Read the model definition and answer for the solid it produces. Units are mm, in the model's axes. A direction names the side the tool comes from. Coordinates: 2 decimals unless noted, no trailing zeros. Order: outer loops, then holes, each group sorted by start corner. A loop starts at its lowest first (then second) coordinate and runs counter-clockwise, first axis right, second up.
Autodesk Inventor part; units mm, degrees
ref_plane "Work Plane1" through (0, 2.6, 0) normal (0, -1, 0) x (1, 0, 0)
ref_plane "YZ Plane" through (0, 0, 0) normal (1, 0, 0) x (0, 1, 0)
ref_plane "XZ Plane" through (0, 0, 0) normal (0, 1, 0) x (-1, 0, 0)
sketch "Sketch1" plane through (0, 0, 0) normal (0, 1, 0) x (-1, 0, 0)
  line L0 (4.7, 5.15) -> (-4.7, 5.15)
  line L1 (-4.7, 5.15) -> (-4.7, -5.15)
  line L2 (-4.7, -5.15) -> (4.7, -5.15)
  line L3 (4.7, -5.15) -> (4.7, 5.15)
  point P0 (0, 0)
  dimension "d0" = 9.4
  dimension "d1" = 4.7
  dimension "d2" = 10.3
  dimension "d3" = 5.15
extrude "Extrusion1" add sketch "Sketch1" along normal blind 4.7
chamfer "Chamfer1" distance 3.3 angle 15 1 edges at (0, 4.7, 5.15) measured on face at (-1.5667, 1.5667, 5.15)
chamfer "Chamfer2" distance 3.3 angle 15 1 edges at (4.7, 4.7, -0.4421) measured on face at (4.7, 3.1333, -2.0114)
chamfer "Chamfer3" distance 3.3 angle 15 1 edges at (-0.4421, 4.7, -5.15) measured on face at (-1.8614, 3.1333, -5.15)
chamfer "Chamfer4" distance 3.3 angle 15 1 edges at (-4.7, 4.7, 0) measured on face at (-4.7, 2.5, -1.4219)
sketch "Sketch2" plane through (0, 0, 0) normal (0, -1, 0) x (1, 0, 0)
  line L0 (4.7, 5.15) -> (4.7, -5.15)
  line L1 (11.3, -5.15) -> (11.3, 5.1662)
  line L2 (11.3, 5.1662) -> (4.7, 5.1662)
  line L3 (4.7, 5.1662) -> (4.7, -5.15)
  line L4 (-4.7, 5.15) -> (4.7, 5.15)
  line L5 (11.3, -5.15) -> (11.3, -5.1902)
  line L6 (11.3, -5.1902) -> (4.7, -5.1902)
  line L7 (4.7, -5.1902) -> (4.7, -5.15)
  point P0 (0, 0)
  dimension "d18" = 6.6
extrude "Extrusion2" add sketch "Sketch2" against normal blind 1.4 and the other way blind 0.01
ref_plane "Work Plane1" through (0, 2.6, 0) normal (0, -1, 0) x (1, 0, 0)
sketch "Sketch3" plane through (0, 2.6, 0) normal (0, -1, 0) x (1, 0, 0)
  line L0 (-4.304, -0.8) -> (-8, -0.8)
  line L1 (-8, -0.8) -> (-8, 0.8)
  line L2 (-8, 0.8) -> (-4.304, 0.8)
  line L3 (-4.304, 0.8) -> (-4.304, -0.8)
  line L4 (-4.7, -5.15) -> (-4.7, 5.15)
  line L5 (-4.7, -5.15) -> (-4.7, 5.15)
  line L6 (-4.7, 0) -> (-3.1889, 0)
  line L7 (-8, -0.45) -> (-7.7, -0.8)
  line L8 (-8, 0.45) -> (-7.7, 0.8)
  point P0 (0, 0)
  dimension "d25" = 3.3
  dimension "d26" = 1.6
  dimension "d27" = 0.8
  dimension "d28" = 3
  dimension "d29" = 3
  dimension "d30" = 0.9
  dimension "d31" = 0.45
extrude "Extrusion3" add sketch "Sketch3" along normal mid plane 0.7 contours L7 L1 L8 L2 L4 L0 | L4 L6 L3 L0 | L4 L2 L3 L6
sketch "Sketch4" plane through (-8, 2.25, -0.45) normal (-1, 0, 0) x (0, 0, 1)
  line L0 (1.25, 0.7) -> (-0.35, 0.7)
  line L1 (1.25, 0) -> (-0.35, 0)
  line L2 (0.9, 0.7) -> (0, 0.7)
  line L3 (0, 0.7) -> (0, 0)
  line L4 (0, 0) -> (0.9, 0)
  line L5 (0.9, 0) -> (0.9, 0.7)
  line L6 (0.9, 0.7) -> (0.9, 0)
  line L7 (0.9, 0.126) -> (0.9, 0.1378)
  point P0 (0.45, -2.25)
  dimension "d34" = 0.9
  dimension "d35" = 0
sketch "Sketch5" plane through (0, 0, 0) normal (0, 0, 1) x (1, 0, 0)
  line L0 (-8, 2.95) -> (-8, 2.25)
  line L1 (-8, 2.6) -> (-8.8, 2.6)
  line L2 (-10.8, 4.6) -> (-10.8, 8.6)
  line L3 (-4.557, 8.6) -> (-13.8977, 8.6)
  line L4 (4.7, 0) -> (-4.7, 0)
  arc A0 (-10.8, 4.6) -> (-8.8, 2.6) centre (-8.8, 4.6) ccw
  point P0 (0, 0)
  dimension "d36" = 8.6
  dimension "d38" = 2.8
  dimension "d39" = 2
sweep "Sweep1" add profiles "Sketch4" path "Sketch5" path curves L1 A0 L2
pattern_linear "Rectangular Pattern1" count 3 spacing 2.54 along (0, 0, -1) of "Extrusion3", "Sweep1" first direction both ways yes
properties part number "TO-220_UnderHeat"
Q1. The part is cut by section A-A, the plane y = 7.5. Determine the outline of the cut face in (x, z), then the cut area to 3 significant figures.
Q2. The part is cut by section C-C, the plane y = 3.25. Determine the outline of the cut face in (x, z).
Q3. The part is cut by section B-B, the plane x = -5.75. Determine the outline of the cut face in (y, z), then the cut area to 3 significant figures.
Q4. Each of these flat-tipped pins is pushed along its axis until it touches: P1, Ø0.8, axis at x = -6, z = 2.5, coming from the -Y side; P2, Ø2, axis at x = -7.5, z = 3.5, coming from the +Y side; P3, Ø3.5, axis at x = 6.5, z = -2, coming from the +Y side; P4, Ø4, axis at x = 3, z = -3.5, coming from the -Y side. Where does it stop, or does it pass through?
Q5. Straight lines are drawn through the part: L1, parallel to Z at x = -9.25, y = 2.75; L2, parallel to Y at x = -3.5, z = -3; L3, parallel to Y at x = 9.5, z = 0.25. For each, find the intervals that lie inside material, in ascending order.
Q6. Determine the mould class of faces 1 (the flat face through (-11, 5, 0.45)), 2 (the flat face through (-7, 2.95, -3)), 3 (the flat face through (11.3, 1, 0)) for opening direction X: +X half, -X half, draft (parallel to the pull), parting line (faces both ways), or undercut.
Q7. Which of the six approach directions +Z, -Z, +X, -X, +Y, -Y give full straight-line access (tool end or side, diameter ignored) to faces 4 (the flat face through (0, 1, 5.15)), 5 (the cylindrical face through (-9.954, 3.421, 2.534)), 6 (the flat face through (8, 1.4, 0)), 7 (the flat face through (-11, 5, -0.45))?
Computed values:
1. outline: (-11.15, -2.99) - (-10.45, -2.99) - (-10.45, -2.09) - (-11.15, -2.09) - close; (-11.15, -0.45) - (-10.45, -0.45) - (-10.45, 0.45) - (-11.15, 0.45) - close; (-11.15, 2.09) - (-10.45, 2.09) - (-10.45, 2.99) - (-11.15, 2.99) - close
1. area: 1.89 mm2
2. outline: (-10.72, -2.99) - (-9.75, -2.99) - (-9.75, -2.09) - (-10.72, -2.09) - close; (-10.72, -0.45) - (-9.75, -0.45) - (-9.75, 0.45) - (-10.72, 0.45) - close; (-10.72, 2.09) - (-9.75, 2.09) - (-9.75, 2.99) - (-10.72, 2.99) - close; (-4.2, -4.65) - (4.2, -4.65) - (4.2, 4.65) - (-4.2, 4.65) - close
3. outline: (2.25, -3.34) - (2.95, -3.34) - (2.95, -1.74) - (2.25, -1.74) - close; (2.25, -0.8) - (2.95, -0.8) - (2.95, 0.8) - (2.25, 0.8) - close; (2.25, 1.74) - (2.95, 1.74) - (2.95, 3.34) - (2.25, 3.34) - close
3. area: 3.36 mm2
4. P1: stops at y = 2.25
4. P2: stops at y = 2.95
4. P3: stops at y = 1.4
4. P4: stops at y = -0.01
5. L1: z = -2.99 to -2.09, -0.45 to 0.45, 2.09 to 2.99
5. L2: y = 0 to 4.7
5. L3: y = -0.01 to 1.4
6. face 1: draft
6. face 2: undercut
6. face 3: +X half
7. face 4: +Z, -X, +Y, -Y
7. face 5: +Z, -Z, +Y
7. face 6: +Z, -Z, +X, +Y
7. face 7: -X, +Y, -Y
